Work out the finished part from the listing and answer in its coordinate system (mm). A direction names the side the tool comes from. Coordinates: 2 decimals unless noted, no trailing zeros. Loops run counter-clockwise (first coordinate to the right, second up) from the corner with the lowest first, then second, coordinate; pieces in that order, holes last. Notation, with made-up numbers: M -28.75,-28 L 23.25,-28 A17 cw 23.25,4 Z; hole C 38,61.25 d5. An arc over 180 degrees is marked long. Write each question's results on one line, items separated by ' | '.
```python
from build123d import *

# Parameters (mm, degrees)
SKETCH_1_R          = 16.75
EXTRUDE_1_DEPTH     = 1
SKETCH_2_R          = 10.35
EXTRUDE_2_DEPTH     = 0.65
SKETCH_3_R          = 5.25
CUT_EXTRUDE_1_DEPTH = 2.65
SKETCH_4_R          = 0.6499985
EXTRUDE_3_DEPTH     = 3.6


with BuildPart() as part:
    # Эскиз1 → Бобышка-Вытянуть1 (new body)
    with BuildSketch(Plane(origin=(0, 0, 0), x_dir=(1, 0, 0), z_dir=(0, 1, 0))):
        Circle(SKETCH_1_R)
    extrude(amount=EXTRUDE_1_DEPTH)

    # Эскиз2 → Бобышка-Вытянуть2 (add)
    with BuildSketch(Plane(origin=(0, 1, 0), x_dir=(1, 0, 0), z_dir=(0, 1, 0))):
        Circle(SKETCH_2_R)
    extrude(amount=EXTRUDE_2_DEPTH)

    # Эскиз3 → Вырез-Вытянуть1 (cut, through all)
    with BuildSketch(Plane(origin=(0, 1.65, 0), x_dir=(1, 0, 0), z_dir=(0, 1, 0))):
        Circle(SKETCH_3_R)
    extrude(amount=-CUT_EXTRUDE_1_DEPTH, mode=Mode.SUBTRACT)

    # Эскиз4 → Бобышка-Вытянуть3 (add)
    with BuildSketch(Plane(origin=(0, 1, 0), x_dir=(1, 0, 0), z_dir=(0, 1, 0))):
        with Locations((14.0000228, 0)):
            Circle(SKETCH_4_R)
        with Locations((-13.999972, 0)):
            Circle(SKETCH_4_R)
    extrude(amount=EXTRUDE_3_DEPTH)


solid = part.part
```
1) Find section A-A, the plane x = 0. Give the vertices of the cut face in (y, z).
Check result:
outline: M 0,-16.75 L 1,-16.75 L 1,-10.35 L 1.65,-10.35 L 1.65,-5.25 L 0,-5.25 Z; M 0,5.25 L 1.65,5.25 L 1.65,10.35 L 1,10.35 L 1,16.75 L 0,16.75 Z
2) Find section D-D, the plane x = 14. Give the vertices of the cut face in (y, z).
Check result:
outline: M 0,-9.2 L 1,-9.2 L 1,-0.65 L 4.6,-0.65 L 4.6,0.65 L 1,0.65 L 1,9.2 L 0,9.2 Z
3) For a pull along Y with two mould halves and no side action, classify faces 1 (the face through (-3.63, 0.49, 16.35)), 2 (the face through (-8, 1, 7)), 3 (the face through (-4, 0, -4)) as released by +Y, released by -Y, zero draft, split by the parting line, or undercut.
Check result:
face 1: zero draft | face 2: released by +Y | face 3: released by -Y
4) Which of the six approach directions +Z, -Z, +X, -X, +Y, -Y give full straight-line access (tool end or side, diameter ignored) to faces 4 (the face through (-14, 4.6, 0)), 5 (the face through (14.6, 2.77, 0.25))?
Check result:
face 4: +Z, -Z, +X, -X, +Y | face 5: +Y
5) Given pin 1 Ø10 at (x, z) = (2.5, 7) entering from +Y; pin 2 Ø5 at (x, z) = (-13.5, 10) entering from +Y, each flat-ended and moving along its own axis, determine where each tip first touches the part or whether it passes through.
Check result:
pin 1: y = 1.65 | pin 2: y = 1
6) Find section B-B, the plane z = 0. Give the vertices of the cut face in (x, y).
Check result:
outline: M -16.75,0 L -5.25,0 L -5.25,1.65 L -10.35,1.65 L -10.35,1 L -13.35,1 L -13.35,4.6 L -14.65,4.6 L -14.65,1 L -16.75,1 Z; M 5.25,0 L 16.75,0 L 16.75,1 L 14.65,1 L 14.65,4.6 L 13.35,4.6 L 13.35,1 L 10.35,1 L 10.35,1.65 L 5.25,1.65 Z
7) Find section C-C, the plane y = 2.15. Give the vertices of the cut face in (x, z), and give its area (3 significant figures).
Check result:
outline: C -14,0 d1.3; C 14,0 d1.3 | area: 2.65 mm^2
8) Straight lines are drawn through the part: probe 1 along X at (y, z) = (1.2, 0); probe 2 along X at (y, z) = (0.8, 0); probe 3 along Z at (x, y) = (0, 1.15). For each, find the intervals that lie inside material, in ascending order. Write a range as [from, to].
Check result:
probe 1: [-14.65, -13.35], [-10.35, -5.25], [5.25, 10.35], [13.35, 14.65] | probe 2: [-16.75, -5.25], [5.25, 16.75] | probe 3: [-10.35, -5.25], [5.25, 10.35]
